Verification items for the finished model (mm, model axes). Give positions to 0.01 mm unless a question says otherwise; leave off trailing zeros. Order: outer loops, then holes, each group sorted by start corner. A loop starts at its lowest first (then second) coordinate and runs counter-clockwise, first axis right, second up.
Autodesk Inventor part; units mm, degrees
ref_plane "YZ Plane" through (0, 0, 0) normal (1, 0, 0) x (0, 1, 0)
ref_plane "XZ Plane" through (0, 0, 0) normal (0, 1, 0) x (-1, 0, 0)
ref_plane "XY Plane" through (0, 0, 0) normal (0, 0, 1) x (1, 0, 0)
sketch "Sketch1" plane through (0, 0, 0) normal (0, 1, 0) x (-1, 0, 0)
  line L0 (0, 0) -> (0, -355.998) construction
  line L1 (5, 0) -> (5, -355.998)
  line L2 (-5, -355.998) -> (-5, 0)
  arc A0 (5, 0) -> (-5, 0) centre (0, 0) ccw
  arc A1 (-5, -355.998) -> (5, -355.998) centre (0, -355.998) ccw
  circle A2 centre (0, 0) radius 1.65
  circle A3 centre (0, -355.998) radius 1.65
  circle A4 centre (0, -57.376) radius 1.65
  point P0 (0, -177.999)
  dimension "d0" = 3.3
  dimension "d1" = 3.3
  dimension "d2" = 10
  dimension "d3" = 355.998
  dimension "d14" = 3.3
  dimension "d15" = 57.376
extrude "Extrusion1" add sketch "Sketch1" along normal blind 3
(1) Section check A-A, the plane x = 0. Enter the section's corners in (y, z).
Solved:
outline: (0, -361) - (3, -361) - (3, -357.65) - (0, -357.65) - close; (0, -354.35) - (3, -354.35) - (3, -59.03) - (0, -59.03) - close; (0, -55.73) - (3, -55.73) - (3, -1.65) - (0, -1.65) - close; (0, 1.65) - (3, 1.65) - (3, 5) - (0, 5) - close
(2) Scan lines: line 1 (Z direction, x = 0, y = 2); line 2 (Z direction, x = 0.25, y = 1.7); line 3 (X direction, y = 1.55, z = -58). Record each from-to range of solid material in increasing order.
Solved:
line 1: z = -361 to -357.65, -354.35 to -59.03, -55.73 to -1.65, 1.65 to 5
line 2: z = -360.99 to -357.63, -354.37 to -59.01, -55.75 to -1.63, 1.63 to 4.99
line 3: x = -5 to -1.53, 1.53 to 5
(3) Go/stop test with a flat-tipped pin: pin 1 (1.5 mm diameter, centred on x = -0.5, y = 1.5, fed in from -Z). Record where the tip stops, or that it passes through.
Solved:
pin 1: stops at z = -361
